Geometry: final body of the model. Coordinates: model frame, mm. Round coordinates to 2 decimals unless told otherwise and drop trailing zeros. Loops run counter-clockwise (first coordinate to the right, second up) from the corner with the lowest first, then second, coordinate; pieces in that order, holes last. Notation, with made-up numbers: (68.5, -15.5) - (121.5, -15.5) arc R17 cw to (121.5, 3.5) - close; hole circle Ø5 at (72, 65.25). An arc over 180 degrees is marked (long way). Use CSV: the item, a comma, the result in double quotes.
Autodesk Fusion 360 part; units mm, degrees
sketch "Skizze1" plane through (0, 0, 0) normal (0, 0, 1) x (1, 0, 0)
  circle A0 centre (0, 0) radius 80
extrude "Extrusion1" add sketch "Skizze1" along normal blind 10 makes body 1
fillet "Abrundung1" radius 2 1 edges at (-74.5862, -28.9292, 10) on bodies 1
sketch "Skizze2" plane through (0, 0, 0) normal (0, 1, 0) x (1, 0, 0)
  line L0 (45, 0) -> (-5, -86.6025) construction
ref_plane "Arbeitsebene1" through (-5, 0, 86.6025) normal (-0.5, 0, 0.866) x (0, -1, 0)
sketch "Skizze3" plane through (-5, 0, 86.6025) normal (-0.5, 0, 0.866) x (0, -1, 0)
  circle A0 centre (0, 0) radius 23
  circle A1 centre (0, 0) radius 20
extrude "Extrusion5" add sketch "Skizze3" against normal blind 110 separate body contours A0 | A1 makes body 2
combine "Kombinieren1" operation add target body 1 tool bodies 2
extrude "Extrusion6" cut sketch "Skizze3" against normal blind 50 bodies 1
fillet "Abrundung2" radius 4 3 edges at (65.7846, 0, 10) (-74.5862, -28.9292, 8) (-72.7215, 28.206, 10) on bodies 1
sketch "Skizze4" plane through (-5, 0, 86.6025) normal (-0.5, 0, 0.866) x (0, -1, 0)
  circle A0 centre (0, 0) radius 15.75
extrude "Extrusion7" cut sketch "Skizze4" against normal blind 110 bodies 1
sketch "Skizze5" plane through (0, 0, 0) normal (0, 0, 1) x (1, 0, 0)
  circle A0 centre (0, 0) radius 160
extrude "Extrusion8" cut sketch "Skizze5" against normal blind 110 bodies 1
sketch "Skizze6" plane through (0, 0, 0) normal (0, 0, 1) x (1, 0, 0)
  line L0 (45, 0) -> (85, 0)
ref_plane "Arbeitsebene2" through (45, 0, 0) normal (1, 0, 0) x (0, 1, 0)
sketch "Skizze7" plane through (45, 0, 0) normal (1, 0, 0) x (0, 1, 0)
  line L0 (-4, 0) -> (-4, 1.7)
  line L1 (-4, 1.7) -> (-3.2, 3.3)
  line L2 (-3.2, 3.3) -> (-1, 5.5)
  line L3 (-1, 5.5) -> (1, 5.5)
  line L4 (1, 5.5) -> (3.2, 3.3)
  line L5 (3.2, 3.3) -> (4, 1.7)
  line L6 (4, 1.7) -> (4, 0)
  line L7 (4, 0) -> (-4, 0)
sweep "Sweeping1" cut profiles "Skizze7" path "Skizze6" along L0 section 1 bodies 1
sketch "Skizze8" plane through (0, 0, 0) normal (0, 0, 1) x (1, 0, 0)
  circle A0 centre (0, 0) radius 72.5
extrude "Extrusion9" cut sketch "Skizze8" along normal blind 3 bodies 1
sketch "Skizze9" plane through (0, 0, 0) normal (0, 0, 1) x (1, 0, 0)
  line L0 (72.2241, -6.3188) -> (73.7184, -6.4495)
  arc A0 (73.7184, -6.4495) -> (73.7184, 6.4495) centre (0, 0) ccw
  line L1 (73.7184, 6.4495) -> (72.2241, 6.3188)
  arc A1 (72.2241, -6.3188) -> (72.2241, 6.3188) centre (0, 0) ccw
  line L2 (6.3188, 72.2241) -> (6.4495, 73.7184)
  arc A2 (6.4495, 73.7184) -> (-6.4495, 73.7184) centre (0, 0) ccw
  line L3 (-6.4495, 73.7184) -> (-6.3188, 72.2241)
  arc A3 (6.3188, 72.2241) -> (-6.3188, 72.2241) centre (0, 0) ccw
  line L4 (-72.2241, 6.3188) -> (-73.7184, 6.4495)
  arc A4 (-73.7184, 6.4495) -> (-73.7184, -6.4495) centre (0, 0) ccw
  line L5 (-73.7184, -6.4495) -> (-72.2241, -6.3188)
  arc A5 (-72.2241, 6.3188) -> (-72.2241, -6.3188) centre (0, 0) ccw
  line L6 (-6.3188, -72.2241) -> (-6.4495, -73.7184)
  arc A6 (-6.4495, -73.7184) -> (6.4495, -73.7184) centre (0, 0) ccw
  line L7 (6.4495, -73.7184) -> (6.3188, -72.2241)
  arc A7 (-6.3188, -72.2241) -> (6.3188, -72.2241) centre (0, 0) ccw
extrude "Extrusion10" cut sketch "Skizze9" along normal blind 3 bodies 1
sketch "Skizze10" plane through (0, 0, 0) normal (0, 0, 1) x (1, 0, 0)
  line L0 (72.2241, -6.3188) -> (73.7184, -6.4495)
  arc A0 (73.7184, -6.4495) -> (69.5373, 25.3095) centre (0, 0) ccw
  line L1 (69.5373, 25.3095) -> (68.1277, 24.7965)
  arc A1 (72.2241, -6.3188) -> (68.1277, 24.7965) centre (0, 0) ccw
  line L2 (6.3188, 72.2241) -> (6.4495, 73.7184)
  arc A2 (6.4495, 73.7184) -> (-25.3095, 69.5373) centre (0, 0) ccw
  line L3 (-25.3095, 69.5373) -> (-24.7965, 68.1277)
  arc A3 (6.3188, 72.2241) -> (-24.7965, 68.1277) centre (0, 0) ccw
  line L4 (-72.2241, 6.3188) -> (-73.7184, 6.4495)
  arc A4 (-73.7184, 6.4495) -> (-69.5373, -25.3095) centre (0, 0) ccw
  line L5 (-69.5373, -25.3095) -> (-68.1277, -24.7965)
  arc A5 (-72.2241, 6.3188) -> (-68.1277, -24.7965) centre (0, 0) ccw
  line L6 (-6.3188, -72.2241) -> (-6.4495, -73.7184)
  arc A6 (-6.4495, -73.7184) -> (25.3095, -69.5373) centre (0, 0) ccw
  line L7 (25.3095, -69.5373) -> (24.7965, -68.1277)
  arc A7 (-6.3188, -72.2241) -> (24.7965, -68.1277) centre (0, 0) ccw
extrude "Extrusion11" cut sketch "Skizze10" along normal blind 1.25 from surface at 1.75 bodies 1
sketch "Skizze11" plane through (0, 0, 0) normal (0, 0, 1) x (1, 0, 0)
  circle A0 centre (0, 0) radius 72.2
extrude "Extrusion12" add sketch "Skizze11" along normal blind 3 separate body makes body 3
fillet "Abrundung3" radius 0.5 1 edges at (-67.314, -26.1086, 3) on bodies 3
sketch "Skizze12" plane through (0, 0, 0) normal (0, 0, 1) x (1, 0, 0)
  line L0 (71.0266, -4.9667) -> (73.5205, -5.1411)
  arc A0 (73.5205, -5.1411) -> (73.5205, 5.1411) centre (0, 0) ccw
  line L1 (73.5205, 5.1411) -> (71.0266, 4.9667)
  arc A1 (71.0266, -4.9667) -> (71.0266, 4.9667) centre (0, 0) ccw
  line L2 (4.9667, 71.0266) -> (5.1411, 73.5205)
  arc A2 (5.1411, 73.5205) -> (-5.1411, 73.5205) centre (0, 0) ccw
  line L3 (-5.1411, 73.5205) -> (-4.9667, 71.0266)
  arc A3 (4.9667, 71.0266) -> (-4.9667, 71.0266) centre (0, 0) ccw
  line L4 (-71.0266, 4.9667) -> (-73.5205, 5.1411)
  arc A4 (-73.5205, 5.1411) -> (-73.5205, -5.1411) centre (0, 0) ccw
  line L5 (-73.5205, -5.1411) -> (-71.0266, -4.9667)
  arc A5 (-71.0266, 4.9667) -> (-71.0266, -4.9667) centre (0, 0) ccw
  line L6 (-4.9667, -71.0266) -> (-5.1411, -73.5205)
  arc A6 (-5.1411, -73.5205) -> (5.1411, -73.5205) centre (0, 0) ccw
  line L7 (5.1411, -73.5205) -> (4.9667, -71.0266)
  arc A7 (-4.9667, -71.0266) -> (4.9667, -71.0266) centre (0, 0) ccw
extrude "Extrusion13" add sketch "Skizze12" along normal blind 1.1 from surface at 1.9 separate body makes body 4 at (72.7424, 3.9409, 1.9) makes body 5 at (-72.7424, 3.9409, 1.9) makes body 6 at (-3.9409, 72.7424, 1.9) makes body 7 at (0.5522, -72.8469, 1.9)
combine "Kombinieren2" operation add target body 3 tool bodies 4 5 6 7
sketch "Skizze13" plane through (0, 0, 0) normal (0, 0, 1) x (1, 0, 0)
  circle A0 centre (0, 39.875) radius 9
  circle A1 centre (0, -39.875) radius 9
extrude "Extrusion14" cut sketch "Skizze13" along normal blind 3 bodies 3
delete_body "Körper entfernen1" bodies 1
equation "base_plate_diameter = 160 mm"
equation "base_plate_height = 10 mm"
equation "base_plate_rounding = 2 mm"
equation "leg_outer_diameter = 46 mm"
equation "ring_inner_diameter = 40 mm"
equation "ring_extrude_depth = 50 mm"
equation "hole_inner_diameter = 31.5 mm"
equation "leg_length = 100 mm"
equation "leg_angle = 120 deg"
equation "leg_offset = 45 mm"
equation "leg_plate_rounding = 4 mm"
equation "cable_channel_width = 8 mm"
equation "cable_channel_depth = 5.5 mm"
equation "cable_channel_vertical_height = 2.5 mm"
equation "cable_channel_edge_chamfer = 0.8 mm"
equation "cover_plate_diameter = 145 mm"
equation "cover_plate_thickness = 3 mm"
equation "finger_grip_diameter = 18 mm"
equation "finger_grip_depth = 1.5 mm"
equation "clamp_recess_width = 22 mm"
equation "clamp_recess_length = 12 mm"
equation "clamp_recess_depth = 2.5 mm"
equation "strain_relief_screw_diameter = 2.6 mm"
equation "strain_relief_screw_depth = 6 mm"
equation "d25 = base_plate_height"
equation "d28 = base_plate_rounding"
equation "d41 = leg_plate_rounding"
equation "d53 = cover_plate_thickness"
equation "d55 = cover_plate_thickness"
equation "d60 = cover_plate_thickness"
equation "d67 = cover_plate_thickness"
Item 1: Material intervals for line 1 (Y direction, x = 0, z = 2.3) (3 decimals); line 2 (Y direction, x = 0, z = 0.8) (3 decimals); line 3 (X direction, y = 43.5, z = 0.3), sorted ascending.
Final values:
line 1,"y = -73.7 to -48.875, -30.875 to 30.875, 48.875 to 73.7"
line 2,"y = -72.2 to -48.875, -30.875 to 30.875, 48.875 to 72.2"
line 3,"x = -57.62 to -8.24, 8.24 to 57.62"
Item 2: Mould query, pull axis Y, two halves, no side actions, for faces 1 (the cylindrical face through (-1.17, 30.95, 1.48)), 2 (the cylindrical face through (66.694, 27.653, 1.232)), 3 (the flat face through (-1, 1, 0)), 4 (the cylindrical face through (4.838, -47.464, 1.479)). Classes: released by +Y, released by -Y, zero draft, split by the parting line, or undercut.
Final values:
face 1,"undercut"
face 2,"split by the parting line"
face 3,"zero draft"
face 4,"undercut"
Item 3: Section A-A on x = 0. Return the cut outline in (y, z) (3 decimals).
Final values:
outline,"(-73.7, 1.9) - (-72.2, 1.9) - (-72.2, 0) - (-48.875, 0) - (-48.875, 3) - (-73.7, 3) - close; (-30.875, 0) - (30.875, 0) - (30.875, 3) - (-30.875, 3) - close; (48.875, 0) - (72.2, 0) - (72.2, 1.9) - (73.7, 1.9) - (73.7, 3) - (48.875, 3) - close"
Item 4: Section B-B on z = 1.2. Return the cut outline in (x, y) (3 decimals), plus the area to 3 significant figures.
Final values:
outline,"circle Ø144.4 at (0, 0); hole circle Ø18 at (0, -39.875); hole circle Ø18 at (0, 39.875)"
area,"15,900 mm²"
Item 5: Pin query (flat end, axial travel): P1, Ø0.5, axis at x = -72.5, y = 2, coming from the -Z side; P2, Ø1.5, axis at y = -26.5, z = 1, coming from the +X side; P3, Ø1, axis at x = -29.5, z = 2.5, coming from the -Y side; P4, Ø11, axis at x = 0, y = -39.875, coming from the +Z side. Return the tip coordinate at first contact, or that it passes through.
Final values:
P1,"stops at z = 1.9"
P2,"stops at x = 67.45"
P3,"stops at y = -66.12"
P4,"passes through"
